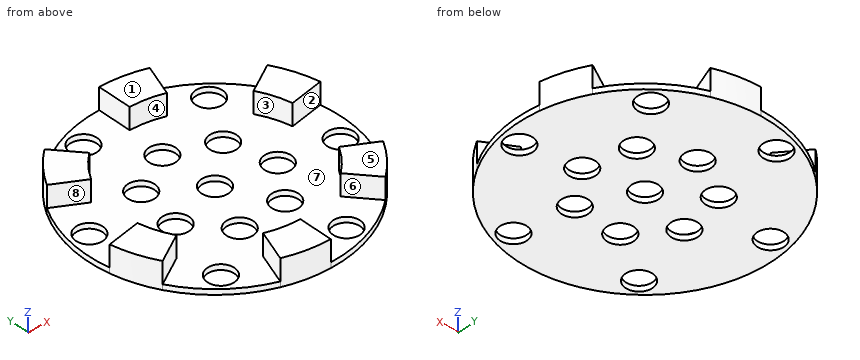
```python
from build123d import *

# Parameters (mm, degrees)
SKETCH1_R           = 5
BOSS_EXTRUDE1_DEPTH = 2
SKETCH1_3_R         = 5
BOSS_EXTRUDE2_DEPTH = 10


with BuildPart() as part:
    # Sketch1 → Boss-Extrude1 (new body)
    with BuildSketch(Plane.XY):
        with BuildLine():
            ThreePointArc((-22.497566339, 26.811555509), (-26.811555509, 22.497566339), (-30.310889132, 17.5))
            Line((-30.310889132, 17.5), (-41.13620668, 23.75))
            ThreePointArc((-41.13620668, 23.75), (-46.778368268, 8.248288439), (-46.778368268, -8.248288439))
            Line((-46.778368268, -8.248288439), (-34.468271355, -6.077686218))
            ThreePointArc((-34.468271355, -6.077686218), (-32.889241728, -11.970705016), (-30.310889132, -17.5))
            Line((-30.310889132, -17.5), (-41.13620668, -23.75))
            ThreePointArc((-41.13620668, -23.75), (-30.53241146, -36.387111048), (-16.245956808, -44.635399487))
            Line((-16.245956808, -44.635399487), (-11.970705016, -32.889241728))
            ThreePointArc((-11.970705016, -32.889241728), (-6.077686218, -34.468271355), (0, -35))
            Line((0, -35), (0, -47.5))
            ThreePointArc((0, -47.5), (16.245956808, -44.635399487), (30.53241146, -36.387111048))
            Line((30.53241146, -36.387111048), (22.497566339, -26.811555509))
            ThreePointArc((22.497566339, -26.811555509), (26.811555509, -22.497566339), (30.310889132, -17.5))
            Line((30.310889132, -17.5), (41.13620668, -23.75))
            ThreePointArc((41.13620668, -23.75), (46.778368268, -8.248288439), (46.778368268, 8.248288439))
            Line((46.778368268, 8.248288439), (34.468271355, 6.077686218))
            ThreePointArc((34.468271355, 6.077686218), (32.889241728, 11.970705016), (30.310889132, 17.5))
            Line((30.310889132, 17.5), (41.13620668, 23.75))
            ThreePointArc((41.13620668, 23.75), (30.53241146, 36.387111048), (16.245956808, 44.635399487))
            Line((16.245956808, 44.635399487), (11.970705016, 32.889241728))
            ThreePointArc((11.970705016, 32.889241728), (6.077686218, 34.468271355), (0, 35))
            Line((0, 35), (0, 47.5))
            ThreePointArc((0, 47.5), (-16.245956808, 44.635399487), (-30.53241146, 36.387111048))
            Line((-30.53241146, 36.387111048), (-22.497566339, 26.811555509))
        make_face()
        with Locations((14.022825876, -38.527397452)):
            Circle(SKETCH1_R, mode=Mode.SUBTRACT)
        with Locations((-26.354291997, -31.407822168)):
            Circle(SKETCH1_R, mode=Mode.SUBTRACT)
        with Locations((40.377117874, -7.119575284)):
            Circle(SKETCH1_R, mode=Mode.SUBTRACT)
        with Locations((-40.377117874, 7.119575284)):
            Circle(SKETCH1_R, mode=Mode.SUBTRACT)
        with Locations((26.354291997, 31.407822168)):
            Circle(SKETCH1_R, mode=Mode.SUBTRACT)
        with Locations((-14.022825876, 38.527397452)):
            Circle(SKETCH1_R, mode=Mode.SUBTRACT)
        with Locations((15.370514661, 13.564559671)):
            Circle(SKETCH1_R, mode=Mode.SUBTRACT)
        with Locations((-7.962913324, -18.890262343)):
            Circle(SKETCH1_R, mode=Mode.SUBTRACT)
        with Locations((-19.733797062, -5.552229597)):
            Circle(SKETCH1_R, mode=Mode.SUBTRACT)
        with Locations((9.804206562, -18.003542254)):
            Circle(SKETCH1_R, mode=Mode.SUBTRACT)
        with Locations((20.188558937, -3.559787642)):
            Circle(SKETCH1_R, mode=Mode.SUBTRACT)
        with Locations((-16.644729117, 11.966745281)):
            Circle(SKETCH1_R, mode=Mode.SUBTRACT)
        with Locations((-1.021840656, 20.474516885)):
            Circle(SKETCH1_R, mode=Mode.SUBTRACT)
        Circle(SKETCH1_R, mode=Mode.SUBTRACT)
    extrude(amount=BOSS_EXTRUDE1_DEPTH)

    # Sketch1_3 → Boss-Extrude2 (add)
    with BuildSketch(Plane.XY):
        with BuildLine():
            ThreePointArc((-30.310889132, 17.5), (-26.811555509, 22.497566339), (-22.497566339, 26.811555509))
            Line((-22.497566339, 26.811555509), (-30.53241146, 36.387111048))
            ThreePointArc((-30.53241146, 36.387111048), (-36.387111048, 30.53241146), (-41.13620668, 23.75))
            Line((-41.13620668, 23.75), (-30.310889132, 17.5))
        make_face()
        with Locations((-31.407822168, 26.354291997)):
            Circle(SKETCH1_3_R, mode=Mode.SUBTRACT)
        with BuildLine():
            ThreePointArc((-30.310889132, -17.5), (-32.889241728, -11.970705016), (-34.468271355, -6.077686218))
            Line((-34.468271355, -6.077686218), (-46.778368268, -8.248288439))
            ThreePointArc((-46.778368268, -8.248288439), (-44.635399487, -16.245956808), (-41.13620668, -23.75))
            Line((-41.13620668, -23.75), (-30.310889132, -17.5))
        make_face()
        with Locations((-38.527397452, -14.022825876)):
            Circle(SKETCH1_3_R, mode=Mode.SUBTRACT)
        with BuildLine():
            ThreePointArc((0, -35), (-6.077686218, -34.468271355), (-11.970705016, -32.889241728))
            Line((-11.970705016, -32.889241728), (-16.245956808, -44.635399487))
            ThreePointArc((-16.245956808, -44.635399487), (-8.248288439, -46.778368268), (0, -47.5))
            Line((0, -47.5), (0, -35))
        make_face()
        with Locations((-7.119575284, -40.377117874)):
            Circle(SKETCH1_3_R, mode=Mode.SUBTRACT)
        with BuildLine():
            Line((41.13620668, -23.75), (30.310889132, -17.5))
            ThreePointArc((30.310889132, -17.5), (26.811555509, -22.497566339), (22.497566339, -26.811555509))
            Line((22.497566339, -26.811555509), (30.53241146, -36.387111048))
            ThreePointArc((30.53241146, -36.387111048), (36.387111048, -30.53241146), (41.13620668, -23.75))
        make_face()
        with Locations((31.407822168, -26.354291997)):
            Circle(SKETCH1_3_R, mode=Mode.SUBTRACT)
        with BuildLine():
            Line((41.13620668, 23.75), (30.310889132, 17.5))
            ThreePointArc((30.310889132, 17.5), (32.889241728, 11.970705016), (34.468271355, 6.077686218))
            Line((34.468271355, 6.077686218), (46.778368268, 8.248288439))
            ThreePointArc((46.778368268, 8.248288439), (44.635399487, 16.245956808), (41.13620668, 23.75))
        make_face()
        with Locations((38.527397452, 14.022825876)):
            Circle(SKETCH1_3_R, mode=Mode.SUBTRACT)
        with BuildLine():
            Line((0, 47.5), (0, 35))
            ThreePointArc((0, 35), (6.077686218, 34.468271355), (11.970705016, 32.889241728))
            Line((11.970705016, 32.889241728), (16.245956808, 44.635399487))
            ThreePointArc((16.245956808, 44.635399487), (8.248288439, 46.778368268), (0, 47.5))
        make_face()
        with Locations((7.119575284, 40.377117874)):
            Circle(SKETCH1_3_R, mode=Mode.SUBTRACT)
        with Locations((7.119575284, 40.377117874)):
            Circle(SKETCH1_3_R)
        with Locations((-31.407822168, 26.354291997)):
            Circle(SKETCH1_3_R)
        with Locations((-38.527397452, -14.022825876)):
            Circle(SKETCH1_3_R)
        with Locations((-7.119575284, -40.377117874)):
            Circle(SKETCH1_3_R)
        with Locations((31.407822168, -26.354291997)):
            Circle(SKETCH1_3_R)
        with Locations((38.527397452, 14.022825876)):
            Circle(SKETCH1_3_R)
    extrude(amount=BOSS_EXTRUDE2_DEPTH)


solid = part.part
```
Check sheet for the modelled part. Datum: model origin and axes. Units: mm. Face numbers are marked on the shaded views. A direction names the side the tool comes from. Coordinates: 2 decimals unless noted, no trailing zeros. Order: outer loops, then holes, each group sorted by start corner. A loop starts at its lowest first (then second) coordinate and runs counter-clockwise, first axis right, second up. Notation, with made-up numbers: (17.25, 41) -> (61.25, 41) arc R9 ccw to (61.25, 49) -> close; hole circle Ø8 at (73.5, 63). An arc over 180 degrees is marked (long way). Write item = value, one per line. Start each with the question number.
1) Cross-section at D-D (x = -40). Enter the section's corners in (y, z).
2) Cross-section at A-A (z = 4). Enter the section's corners in (x, y).
3) Cross-section at B-B (x = 39). Enter the section's corners in (y, z).
4) Mould release check, pull along Y, two halves, no side actions. Record for the marked faces 1, 2, 3 and 4: +Y half, -Y half, draft (parallel to the pull), parting line (faces both ways), or undercut.
5) Access from +Z, -Z, +X, -X, +Y, -Y to the whole of each face (thin tool, end or side, straight path). Record for the marked faces 5, 6, 7 and 8.
6) Go/stop test with flat-tipped pins: P1, Ø5, axis at x = 13, z = 3, coming from the +Y side; P2, Ø13, axis at x = -7.96, y = -18.89, coming from the +Z side; P3, Ø5, axis at x = -29, y = -16.5, coming from the -Z side; P4, Ø5, axis at y = -25.5, z = 7, coming from the -X side. Record where each tip stops, or that it passes through.
7) Material ranges on L1, parallel to Y at x = 0, z = 1.25; L2, parallel to Z at x = -35.5, y = -2.5; L3, parallel to X at y = -11, z = 0.75, recorded low to high.
8) Cross-section at C-C (y = -15.5). Enter the section's corners in (x, z), then the cut area to 3 significant figures.
Ans:
q1.outline = (-25.62, 0) -> (2.13, 0) -> (2.13, 2) -> (-7.05, 2) -> (-7.05, 10) -> (-23.09, 10) -> (-23.09, 2) -> (-25.62, 2) -> close; (12.11, 0) -> (25.62, 0) -> (25.62, 10) -> (23.09, 10) -> (23.09, 2) -> (12.11, 2) -> close
q2.outline = (-46.78, -8.25) arc R47.5 ccw to (-41.14, -23.75) -> (-30.31, -17.5) arc R35 cw to (-34.47, -6.08) -> close; (-41.14, 23.75) -> (-30.31, 17.5) arc R35 cw to (-22.5, 26.81) -> (-30.53, 36.39) arc R47.5 ccw to start; (-16.25, -44.64) arc R47.5 ccw to (0, -47.5) -> (0, -35) arc R35 cw to (-11.97, -32.89) -> close; (0, 35) arc R35 cw to (11.97, 32.89) -> (16.25, 44.64) arc R47.5 ccw to (0, 47.5) -> close; (22.5, -26.81) -> (30.53, -36.39) arc R47.5 ccw to (41.14, -23.75) -> (30.31, -17.5) arc R35 cw to start; (30.31, 17.5) arc R35 cw to (34.47, 6.08) -> (46.78, 8.25) arc R47.5 ccw to (41.14, 23.75) -> close
q3.outline = (-27.12, 0) -> (-11.93, 0) -> (-11.93, 2) -> (-22.52, 2) -> (-22.52, 10) -> (-27.12, 10) -> close; (-2.31, 0) -> (27.12, 0) -> (27.12, 2) -> (22.52, 2) -> (22.52, 10) -> (6.88, 10) -> (6.88, 2) -> (-2.31, 2) -> close
q4.face_1 = draft
q4.face_2 = undercut
q4.face_3 = undercut
q4.face_4 = -Y half
q5.face_5 = +Z, +X, -X, +Y, -Y
q5.face_6 = +Z, -Y
q5.face_7 = +Z
q5.face_8 = +Z, -X
q6.P1 = 46.32
q6.P2 = 2
q6.P3 = 0
q6.P4 = -41.56
q7.L1 = -47.5 to -5, 5 to 15.58, 25.37 to 47.5
q7.L2 = 0 to 2
q7.L3 = -46.21 to 37.22, 43.53 to 46.21
q8.outline = (-44.9, 0) -> (-11.64, 0) -> (-11.64, 2) -> (-31.38, 2) -> (-31.38, 10) -> (-44.9, 10) -> close; (-4.29, 0) -> (5.48, 0) -> (5.48, 2) -> (-4.29, 2) -> close; (14.13, 0) -> (44.9, 0) -> (44.9, 2) -> (14.13, 2) -> close
q8.area = 256 mm²
